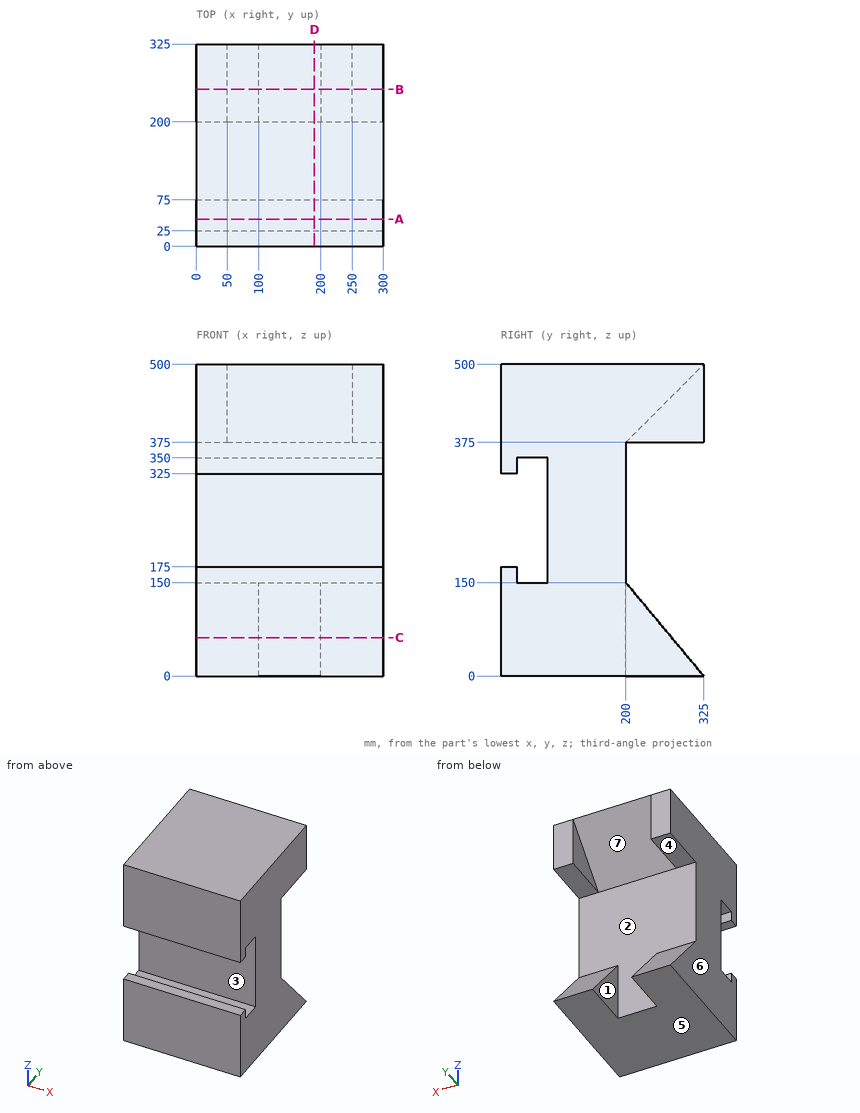
Study the drawing (mm; zero at the part's minimum x, y, z) and answer. A direction names the side the tool comes from. Coordinates: 2 decimals unless noted, no trailing zeros. Write each loop counter-clockwise with the first axis right and the second up, starting at its lowest first coordinate (ties: lowest second). Pieces come first, ordered by that corner, then holes. Notation, with made-up numbers: (80.5, -36.75) - (95.5, -36.75) arc R13 cw to (95.5, -27.75) - close; hole circle Ø1 at (-20, -23.5). An arc over 180 degrees is marked (long way). Put each result on its own line as item: value.
1. Find the intervals of material crossed by line 1 along Z through (x, y) = (109, 63.5); line 2 along Y through (x, z) = (147.5, 163); line 3 along Y through (x, z) = (106, 308.5), in increasing order. Write a range as from..to.
Answer sheet:
line 1: z = 0..150, 350..500
line 2: y = 0..25, 75..200
line 3: y = 75..200
2. Flat-ended cylindrical pins translate along their axes: pin 1 Ø4 at (x, y) = (141.5, 234) entering from -Z; pin 2 Ø7.5 at (x, z) = (169, 167) entering from +Y. Find the tip coordinate at first contact, or state that the pin passes through.
Answer sheet:
pin 1: stops at z = 407
pin 2: stops at y = 200
3. A tool of negligible diameter and unlimited length cuts with its end or side. For the marked faces 1, 2, 3 and 4, from which of +Z, -Z, +X, -X, +Y, -Y can it reach the whole face along a straight path? Write none if from no direction.
Answer sheet:
face 1: -Z, +Y
face 2: +Y
face 3: +X, -X
face 4: +X, -X, +Y
4. The part is cut by section A-A on y = 44. Give the vertices of the cut face in (x, z).
Answer sheet:
outline: (0, 0) - (300, 0) - (300, 150) - (0, 150) - close; (0, 350) - (300, 350) - (300, 500) - (0, 500) - close
5. The part is cut by section B-B on y = 252. Give the vertices of the cut face in (x, z).
Answer sheet:
outline: (0, 0) - (100, 0) - (100, 87.6) - (0, 87.6) - close; (0, 375) - (50, 375) - (50, 427) - (250, 427) - (250, 375) - (300, 375) - (300, 500) - (0, 500) - close; (200, 0) - (300, 0) - (300, 87.6) - (200, 87.6) - close
6. The part is cut by section D-D on x = 189.5. Give the vertices of the cut face in (y, z).
Answer sheet:
outline: (0, 0) - (200, 0) - (200, 375) - (325, 500) - (0, 500) - (0, 325) - (25, 325) - (25, 350) - (75, 350) - (75, 150) - (25, 150) - (25, 175) - (0, 175) - close
7. The part is cut by section C-C on z = 61.5. Give the vertices of the cut face in (x, y), plus the area to 4 significant figures.
Answer sheet:
outline: (0, 0) - (300, 0) - (300, 273.75) - (200, 273.75) - (200, 200) - (100, 200) - (100, 273.75) - (0, 273.75) - close
area: 74,750 mm^2
8. Determine the mould class of the marked faces 5, 6 and 7 for opening direction X: pulls with the +X half, pulls with the -X half, needs draft (parallel to the pull), parting line crosses it, or undercut.
Answer sheet:
face 5: needs draft
face 6: pulls with the -X half
face 7: undercut
